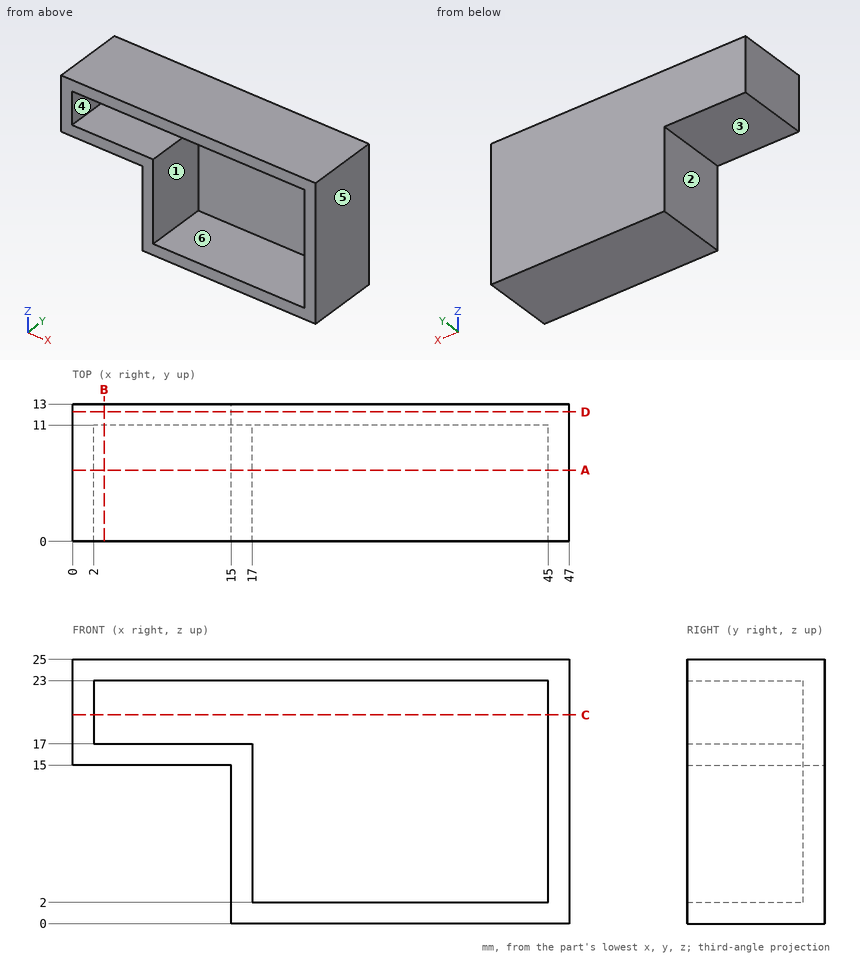
Here's the drawing with two shaded views (mm, measured from the low corner). I have some questions. A direction names the side the tool comes from. Coordinates: 2 decimals unless noted, no trailing zeros. Write each loop counter-clockwise with the first axis right and the second up, starting at its lowest first coordinate (ties: lowest second). Pieces come first, ordered by that corner, then holes. Notation, with made-up numbers: (-16, 47.25) -> (39, 47.25) arc R15 cw to (39, 70.25) -> close; hole circle Ø6 at (62, -14). An arc over 180 degrees is marked (long way). Write item = value, one per line. Start each with the question number.
(1) Will these pins go through, and if not, where does the flat tip stop? pin 1 (1 mm diameter, centred on x = 41.5, z = 22, fed in from -Y); pin 2 (4 mm diameter, centred on x = 8.5, y = 9, fed in from -Z).
(2) I want a section at A-A (y = 6.75). Please give me the cut outline in (x, z).
(3) We'd pull the mould along X, two halves only. Please class the marked faces 1, 2, 3 and 4: released by +X, released by -X, zero draft, split by the parting line, or undercut.
(4) I want a section at B-B (x = 3). Please give me the cut outline in (y, z).
(5) I want a section at C-C (z = 19.75). Please give me the cut outline in (x, y).
(6) I need wall thicknesses on line 1 (Z direction, x = 24.5, y = 5); line 2 (X direction, y = 4, z = 21.75); line 3 (X direction, y = 5.25, z = 8.5). Which ranges of each line are inside material? Lowest first, please. Write a range as [from, to].
(7) I want a section at D-D (y = 12.25). Please give me the cut outline in (x, z), plus the area to 3 significant figures.
(8) Which directions (+Z, -Z, +X, -X, +Y, -Y) give clear straight access to the entire face, cutting with the end or side of a thin tool? Please do the marked faces 5 and 6.
Result set:
q1.pin_1 = 11
q1.pin_2 = 15
q2.outline = (0, 15) -> (15, 15) -> (15, 0) -> (47, 0) -> (47, 25) -> (0, 25) -> close; hole (2, 17) -> (17, 17) -> (17, 2) -> (45, 2) -> (45, 23) -> (2, 23) -> close
q3.face_1 = undercut
q3.face_2 = released by -X
q3.face_3 = zero draft
q3.face_4 = undercut
q4.outline = (0, 15) -> (13, 15) -> (13, 25) -> (0, 25) -> (0, 23) -> (11, 23) -> (11, 17) -> (0, 17) -> close
q5.outline = (0, 0) -> (2, 0) -> (2, 11) -> (45, 11) -> (45, 0) -> (47, 0) -> (47, 13) -> (0, 13) -> close
q6.line_1 = [0, 2], [23, 25]
q6.line_2 = [0, 2], [45, 47]
q6.line_3 = [15, 17], [45, 47]
q7.outline = (0, 15) -> (15, 15) -> (15, 0) -> (47, 0) -> (47, 25) -> (0, 25) -> close
q7.area = 950 mm2
q8.face_5 = +Z, -Z, +X, +Y, -Y
q8.face_6 = -Y
